from build123d import *

# Parameters (mm, degrees)
F0_W     = 44.2
F0_H     = 34.6
F0_W_2   = 39.8
F0_H_2   = 30.2
F1_DEPTH = 2.4
F2_R     = 1
F3_R     = 0.5


with BuildPart() as f1:
    # F0 (on Top) → F1 (new body)
    with BuildSketch(Plane.XY):
        Rectangle(F0_W, F0_H)
        Rectangle(F0_W_2, F0_H_2, mode=Mode.SUBTRACT)
    extrude(amount=F1_DEPTH)

    # F2
    f2_edges = [f1.edges().sort_by_distance(p)[0] for p in [
        (22.1, -17.3, 1.2),
        (19.9, -15.1, 1.2),
        (-22.1, -17.3, 1.2),
        (19.9, 15.1, 1.2),
        (-22.1, 17.3, 1.2),
        (-19.9, 15.1, 1.2),
        (-19.9, -15.1, 1.2),
        (22.1, 17.3, 1.2),
    ]]
    fillet(f2_edges, radius=F2_R)

    # F3
    f3_edges = [f1.edges().sort_by_distance(p)[0] for p in [
        (22.1, 0, 2.4),
        (21.807107, -17.007107, 2.4),
        (21.807107, 17.007107, 2.4),
        (0, -17.3, 2.4),
        (0, 17.3, 2.4),
        (-21.807107, -17.007107, 2.4),
        (-21.807107, 17.007107, 2.4),
        (-22.1, 0, 2.4),
        (-19.9, 0, 2.4),
        (-19.607107, -14.807107, 2.4),
        (-19.607107, 14.807107, 2.4),
        (0, -15.1, 2.4),
        (0, 15.1, 2.4),
        (19.607107, -14.807107, 2.4),
        (19.607107, 14.807107, 2.4),
        (19.9, 0, 2.4),
        (22.1, 0, 0),
        (21.807107, -17.007107, 0),
        (21.807107, 17.007107, 0),
        (0, -17.3, 0),
        (0, 17.3, 0),
        (-21.807107, -17.007107, 0),
        (-21.807107, 17.007107, 0),
        (-22.1, 0, 0),
        (-19.9, 0, 0),
        (-19.607107, -14.807107, 0),
        (-19.607107, 14.807107, 0),
        (0, -15.1, 0),
        (0, 15.1, 0),
        (19.607107, -14.807107, 0),
        (19.607107, 14.807107, 0),
        (19.9, 0, 0),
    ]]
    fillet(f3_edges, radius=F3_R)


solid = f1.part
The model under review builds one solid part; all positions refer to its coordinate system, in mm. A direction names the side the tool comes from. Round coordinates to 2 decimals unless told otherwise and drop trailing zeros. Loops run counter-clockwise (first coordinate to the right, second up) from the corner with the lowest first, then second, coordinate; pieces in that order, holes last. Notation, with made-up numbers: (64.5, -2) -> (92.5, -2) arc R31 cw to (92.5, 29) -> close; hole circle Ø5 at (86.25, 76.5). An arc over 180 degrees is marked (long way). Return JSON: item names as keys, results as strings.
(1) Add section B-B on x = -10. Write out the cut boundary in (y, z), plus the area to 3 significant figures.
Solved:
{"outline": "(-17.3, 0.5) arc R0.5 ccw to (-16.8, 0) -> (-15.6, 0) arc R0.5 ccw to (-15.1, 0.5) -> (-15.1, 1.9) arc R0.5 ccw to (-15.6, 2.4) -> (-16.8, 2.4) arc R0.5 ccw to (-17.3, 1.9) -> close; (15.1, 0.5) arc R0.5 ccw to (15.6, 0) -> (16.8, 0) arc R0.5 ccw to (17.3, 0.5) -> (17.3, 1.9) arc R0.5 ccw to (16.8, 2.4) -> (15.6, 2.4) arc R0.5 ccw to (15.1, 1.9) -> close", "area": "10.1 mm2"}
(2) Add section A-A on y = -10.5. Write out the cut boundary in (x, z), plus the area to 3 significant figures.
Solved:
{"outline": "(-22.1, 0.5) arc R0.5 ccw to (-21.6, 0) -> (-20.4, 0) arc R0.5 ccw to (-19.9, 0.5) -> (-19.9, 1.9) arc R0.5 ccw to (-20.4, 2.4) -> (-21.6, 2.4) arc R0.5 ccw to (-22.1, 1.9) -> close; (19.9, 0.5) arc R0.5 ccw to (20.4, 0) -> (21.6, 0) arc R0.5 ccw to (22.1, 0.5) -> (22.1, 1.9) arc R0.5 ccw to (21.6, 2.4) -> (20.4, 2.4) arc R0.5 ccw to (19.9, 1.9) -> close", "area": "10.1 mm2"}
(3) For line 1 (Y direction, x = 2.5, z = 1.15); line 2 (X direction, y = 12.5, z = 0.7); line 3 (Y direction, x = 5, z = 0.15), list the stretches that pass through material, from the lowest coordinate up.
Solved:
{"line 1": "-17.3 to -15.1, 15.1 to 17.3", "line 2": "-22.1 to -19.9, 19.9 to 22.1", "line 3": "-17.16 to -15.24, 15.24 to 17.16"}
(4) The part is to be moulded in two halves that separate along X. For faces 3 (the cylindrical face through (21.799, 17.015, 1.21)), 4 (the flat face through (0, 15.1, 1)), 5 (the flat face through (-22.1, 0, 1)), 6 (the flat face through (0, -15.1, 1)), say which applies: released by +X, released by -X, zero draft, split by the parting line, or undercut.
Solved:
{"face 3": "released by +X", "face 4": "undercut", "face 5": "released by -X", "face 6": "undercut"}
(5) For faces 1 (the flat face through (-19.9, 0, 1)), 2 (the cylindrical face through (-21.815, -16.999, 1.21)), list the 3-axis set-ups (+Z, -Z, +X, -X, +Y, -Y) from which the entire face can be reached by the end or side of a thin tool; tool diameter is ignored.
Solved:
{"face 1": "+Z, -Z", "face 2": "+Z, -Z, -X, -Y"}
(6) For pin 1 (10 mm diameter, centred on x = 7, y = -10.5, fed in from -Z); pin 2 (8 mm diameter, centred on x = -6, y = 9.5, fed in from -Z), all flat-tipped, find the tip position at first contact; note any pin that passes through.
Solved:
{"pin 1": "z = 0.01", "pin 2": "through"}
(7) Add section C-C on z = 1.15. Write out the cut boundary in (x, y), plus the area to 3 significant figures.
Solved:
{"outline": "(-22.1, -16.3) arc R1 ccw to (-21.1, -17.3) -> (21.1, -17.3) arc R1 ccw to (22.1, -16.3) -> (22.1, 16.3) arc R1 ccw to (21.1, 17.3) -> (-21.1, 17.3) arc R1 ccw to (-22.1, 16.3) -> close; hole (-19.9, -14.1) arc R1 ccw to (-18.9, -15.1) -> (18.9, -15.1) arc R1 ccw to (19.9, -14.1) -> (19.9, 14.1) arc R1 ccw to (18.9, 15.1) -> (-18.9, 15.1) arc R1 ccw to (-19.9, 14.1) -> close", "area": "327 mm2"}
